```python
from build123d import *

# Parameters (mm, degrees)
SKETCH1_W           = 60
SKETCH1_H           = 36
BOSS_EXTRUDE1_DEPTH = 6
SKETCH2_W           = 15
SKETCH2_H           = 6
CUT_EXTRUDE1_DEPTH  = 6
SKETCH3_W           = 6
SKETCH3_H           = 10
CUT_EXTRUDE2_DEPTH  = 6
SKETCH4_R           = 2.5
CUT_EXTRUDE3_DEPTH  = 6


with BuildPart() as part:
    # Sketch1 → Boss-Extrude1 (new body)
    with BuildSketch(Plane.XY):
        with Locations((30, 18)):
            Rectangle(SKETCH1_W, SKETCH1_H)
    extrude(amount=BOSS_EXTRUDE1_DEPTH)

    # Sketch2 → Cut-Extrude1 (cut)
    with BuildSketch(Plane.XY.offset(6)):
        with Locations((7.5, 3)):
            Rectangle(SKETCH2_W, SKETCH2_H)
        with Locations((52.5, 3)):
            Rectangle(SKETCH2_W, SKETCH2_H)
    extrude(amount=-CUT_EXTRUDE1_DEPTH, mode=Mode.SUBTRACT)

    # Sketch3 → Cut-Extrude2 (cut)
    with BuildSketch(Plane.XY.offset(6)):
        with Locations((3, 31)):
            Rectangle(SKETCH3_W, SKETCH3_H)
        with Locations((57, 31)):
            Rectangle(SKETCH3_W, SKETCH3_H)
    extrude(amount=-CUT_EXTRUDE2_DEPTH, mode=Mode.SUBTRACT)

    # Sketch4 → Cut-Extrude3 (cut)
    with BuildSketch(Plane.XY.offset(6)):
        with Locations((30, 21)):
            Circle(SKETCH4_R)
    extrude(amount=-CUT_EXTRUDE3_DEPTH, mode=Mode.SUBTRACT)


solid = part.part
```
The model under review builds one solid part; all positions refer to its coordinate system, in mm. A direction names the side the tool comes from. Give positions to 0.01 mm unless a question says otherwise; leave off trailing zeros. Write each loop counter-clockwise with the first axis right and the second up, starting at its lowest first coordinate (ties: lowest second). Pieces come first, ordered by that corner, then holes. Notation, with made-up numbers: (29, 5.5) -> (40, 5.5) arc R16 cw to (40, 16.5) -> close; hole circle Ø2 at (41.5, 20). An arc over 180 degrees is marked (long way). Answer in a Markdown table with one row per item.
1) Add section B-B on z = 1.45. State the section outline as (x, y) points, plus the area to 3 significant figures.
Worked answers:
| item | result |
|---|---|
| outline | (0, 6) -> (15, 6) -> (15, 0) -> (45, 0) -> (45, 6) -> (60, 6) -> (60, 26) -> (54, 26) -> (54, 36) -> (6, 36) -> (6, 26) -> (0, 26) -> close; hole circle Ø5 at (30, 21) |
| area | 1,840 mm² |
2) Add section C-C on y = 21. State the section outline as (x, z) points, plus the area to 3 significant figures.
Worked answers:
| item | result |
|---|---|
| outline | (0, 0) -> (27.5, 0) -> (27.5, 6) -> (0, 6) -> close; (32.5, 0) -> (60, 0) -> (60, 6) -> (32.5, 6) -> close |
| area | 330 mm² |
3) Add section D-D on y = 2.5. State the section outline as (x, z) points, plus the area to 3 significant figures.
Worked answers:
| item | result |
|---|---|
| outline | (15, 0) -> (45, 0) -> (45, 6) -> (15, 6) -> close |
| area | 180 mm² |
4) Tool access review of faces 4 (the flat face through (54, 31, 3)), 5 (the flat face through (7, 6, 3)), 6 (the flat face through (3, 26, 3)), 7 (the flat face through (52, 6, 3)): name each direction out of +Z, -Z, +X, -X, +Y, -Y from which nothing blocks a thin tool from reaching the whole face with its end or side.
Worked answers:
| item | result |
|---|---|
| face 4 | +Z, -Z, +X, +Y |
| face 5 | +Z, -Z, -X, -Y |
| face 6 | +Z, -Z, -X, +Y |
| face 7 | +Z, -Z, +X, -Y |
5) Clearance check with flat-ended pins moving along their axes: P1, Ø3, axis at y = 2, z = 2, coming from the +X side; P2, Ø1.8, axis at x = 6.5, z = 2.5, coming from the -Y side; P3, Ø3, axis at x = 3, z = 2.5, coming from the +Y side. State where each tip first meets the part, or that it passes through.
Worked answers:
| item | result |
|---|---|
| P1 | x = 45 |
| P2 | y = 6 |
| P3 | y = 26 |
6) Mouldability with a two-part tool opening along X and no side actions: class faces 1 (the flat face through (30, 18, 6)), 2 (the cylindrical face through (29.67, 23.48, 3.04)), 3 (the flat face through (15, 3, 3)) as +X half, -X half, draft (parallel to the pull), parting line (faces both ways), or undercut.
Worked answers:
| item | result |
|---|---|
| face 1 | draft |
| face 2 | undercut |
| face 3 | -X half |
7) For L1, parallel to Y at x = 30, z = 3.55; L2, parallel to X at y = 28, z = 1.1; L3, parallel to Y at x = 49, z = 1.3, list the stretches that pass through material, from the lowest coordinate up. Write a range as [from, to].
Worked answers:
| item | result |
|---|---|
| L1 | [0, 18.5], [23.5, 36] |
| L2 | [6, 54] |
| L3 | [6, 36] |
8) Add section A-A on x = 30. State the section outline as (y, z) points, plus the area to 3 significant figures.
Worked answers:
| item | result |
|---|---|
| outline | (0, 0) -> (18.5, 0) -> (18.5, 6) -> (0, 6) -> close; (23.5, 0) -> (36, 0) -> (36, 6) -> (23.5, 6) -> close |
| area | 186 mm² |
